from build123d import *

# Parameters (mm, degrees)
PROFILEBOSS_EXTRUDE1_DEPTH        = 16
MICROSWITCHHOLESKETCH3_W          = 12.85
MICROSWITCHHOLESKETCH3_H          = 12.05
MICROSWITCHHOLECUT_EXTRUDE1_DEPTH = 2.8
MICROSWITCHHOLESKETCH4_R          = 1.5
MICROSWITCHHOLECUT_EXTRUDE2_DEPTH = 3
CLAMPHOLECUT_EXTRUDE4_REACH       = 38.932
CLAMPHOLESSKETCH6_R               = 2
LONGWIRECHANNELCUT_EXTRUDE5_DEPTH = 37.932370625
CUT_EXTRUDE6_DEPTH                = 2.8
FILLET1_R                         = 2.2
FILLET2_R                         = 2.2


with BuildPart() as part:
    # ProfileSketch2 → ProfileBoss-Extrude1 (new body)
    with BuildSketch(Plane(origin=(0, 0, 0), x_dir=(1, 0, 0), z_dir=(0, 1, 0))):
        Polygon((0, 0), (0, -18), (28, -18), (28, 0), (24, 0), (24, -12), (8, -12), (8, 0), align=None)
    extrude(amount=PROFILEBOSS_EXTRUDE1_DEPTH)

    # MicroSwitchHoleSketch3 → MicroSwitchHoleCut-Extrude1 (cut)
    with BuildSketch(Plane.ZY):
        with Locations((9, 9.975)):
            Rectangle(MICROSWITCHHOLESKETCH3_W, MICROSWITCHHOLESKETCH3_H)
    extrude(amount=-MICROSWITCHHOLECUT_EXTRUDE1_DEPTH, mode=Mode.SUBTRACT)

    # MicroSwitchHoleSketch4 → MicroSwitchHoleCut-Extrude2 (cut)
    with BuildSketch(Plane.ZY.offset(-2.8)):
        with Locations((5.825, 10.95)):
            Circle(MICROSWITCHHOLESKETCH4_R)
        with Locations((12.175, 10.95)):
            Circle(MICROSWITCHHOLESKETCH4_R)
    extrude(amount=-MICROSWITCHHOLECUT_EXTRUDE2_DEPTH, mode=Mode.SUBTRACT)

    # ClampHolesSketch6 → ClampHoleCut-Extrude4 (cut, up to next)
    with BuildSketch(Plane(origin=(28, 0, 0), x_dir=(0, 0, -1), z_dir=(1, 0, 0)), mode=Mode.PRIVATE) as clampholecut_extrude4_sk1:
        with Locations((-9, 12)):
            Circle(CLAMPHOLESSKETCH6_R)
    clampholecut_extrude4_tool1 = extrude(clampholecut_extrude4_sk1.sketch, amount=-CLAMPHOLECUT_EXTRUDE4_REACH, mode=Mode.PRIVATE) & part.part
    # ClampHolesSketch6 → ClampHoleCut-Extrude4 (cut, up to next)
    with BuildSketch(Plane(origin=(28, 0, 0), x_dir=(0, 0, -1), z_dir=(1, 0, 0)), mode=Mode.PRIVATE) as clampholecut_extrude4_sk2:
        with Locations((-9, 4)):
            Circle(CLAMPHOLESSKETCH6_R)
    clampholecut_extrude4_tool2 = extrude(clampholecut_extrude4_sk2.sketch, amount=-CLAMPHOLECUT_EXTRUDE4_REACH, mode=Mode.PRIVATE) & part.part
    add(clampholecut_extrude4_tool1.solids().sort_by_distance((28, 12, 9))[0], mode=Mode.SUBTRACT)
    add(clampholecut_extrude4_tool2.solids().sort_by_distance((28, 4, 9))[0], mode=Mode.SUBTRACT)

    # LongWireChannelSketch7 → LongWireChannelCut-Extrude5 (cut, through all)
    with BuildSketch(Plane.ZY):
        Polygon((18, 2.525), (16.8, 2.525), (16.8, 3.075), (15.6, 3.075), (15.6, 0.875), (16.8, 0.875), (16.8, 1.425), (18, 1.425), align=None)
    extrude(amount=-LONGWIRECHANNELCUT_EXTRUDE5_DEPTH, mode=Mode.SUBTRACT)

    # ShortWireChannelSketch8 → Cut-Extrude6 (cut)
    with BuildSketch(Plane.ZY):
        Polygon((7.9, 3.95), (7.9, 0.875), (15.6, 0.875), (15.6, 3.075), (10.1, 3.075), (10.1, 3.95), align=None)
    extrude(amount=-CUT_EXTRUDE6_DEPTH, mode=Mode.SUBTRACT)

    # Fillet1
    fillet1_edges = [part.edges().sort_by_distance(p)[0] for p in [
        (2.8, 1.975, 15.6),
    ]]
    fillet(fillet1_edges, radius=FILLET1_R)

    # Fillet2
    fillet2_edges = [part.edges().sort_by_distance(p)[0] for p in [
        (28, 1.975, 15.6),
    ]]
    fillet(fillet2_edges, radius=FILLET2_R)


solid = part.part
Model file for the job. Use its own axes, mm. A direction names the side the tool comes from. Give positions to 0.01 mm unless a question says otherwise; leave off trailing zeros. Loops run counter-clockwise (first coordinate to the right, second up) from the corner with the lowest first, then second, coordinate; pieces in that order, holes last.
Item 1: Slice it at C-C (x = 20.75). Write the cut outline in (y, z) (3 decimals), plus the area to 3 significant figures.
Check values:
outline: (0, 12) - (16, 12) - (16, 18) - (2.525, 18) - (2.525, 16.8) - (3.075, 16.8) - (3.075, 15.6) - (0.875, 15.6) - (0.875, 16.8) - (1.425, 16.8) - (1.425, 18) - (0, 18) - close
area: 92.0 mm2
Item 2: Drill centre lines: line 1 along Y through (x, z) = (26.1, 9); line 2 along X through (y, z) = (6, 3.5); line 3 along X through (y, z) = (1.25, 6.75). Where is each one in solid material? Low to high.
Check values:
line 1: y = 0 to 2, 6 to 10, 14 to 16
line 2: x = 2.8 to 8, 24 to 28
line 3: x = 0 to 8, 24 to 28
Item 3: Slice it at A-A (z = 9). Write the cut outline in (x, y) (3 decimals), plus the area to 3 significant figures.
Check values:
outline: (0, 0) - (8, 0) - (8, 16) - (2.8, 16) - (2.8, 0.875) - (0, 0.875) - close; (24, 0) - (28, 0) - (28, 2) - (24, 2) - close; (24, 6) - (28, 6) - (28, 10) - (24, 10) - close; (24, 14) - (28, 14) - (28, 16) - (24, 16) - close
area: 118 mm2
Item 4: Drop flat-ended pins along their axis: P1, Ø2.5, axis at y = 12, z = 9, coming from the -X side; P2, Ø2, axis at x = 14.5, y = 12, coming from the -Z side; P3, Ø1.4, axis at x = 1, z = 5, coming from the +Y side. Give the stop position or say it passes through.
Check values:
P1: stops at x = 2.8
P2: stops at z = 12
P3: stops at y = 3.95
Item 5: Slice it at D-D (z = 5). Write the cut outline in (x, y), plus the area to 3 significant figures.
Check values:
outline: (0, 0) - (8, 0) - (8, 16) - (2.8, 16) - (2.8, 12.2) - (5.8, 12.2) - (5.8, 9.7) - (2.8, 9.7) - (2.8, 3.95) - (0, 3.95) - close; (24, 0) - (28, 0) - (28, 16) - (24, 16) - close
area: 151 mm2
Item 6: Which spindle directions (+Z, -Z, +X, -X, +Y, -Y) get a long thin tool onto all of the face, cutting with end or side? Do faces 4 (the face through (14, 2.525, 17)), 5 (the face through (4.279, 10.375, 13.561)), 6 (the face through (1, 2, 7.9)), 7 (the face through (26, 2, 9)). Say none if no direction does.
Check values:
face 4: +Z, +X, -X
face 5: -X
face 6: -X, +Y
face 7: +X
Item 7: Mould opens along X. For faces 1 (the face through (26, 14, 9)), 2 (the face through (5.8, 11, 6)), 3 (the face through (24, 8, 6)) say: +X half, -X half, draft (parallel to the pull), parting line (faces both ways), or undercut.
Check values:
face 1: draft
face 2: -X half
face 3: undercut
Item 8: Slice it at B-B (y = 10.95). Write the cut outline in (x, z) (3 decimals), plus the area to 3 significant figures.
Check values:
outline: (0, 0) - (8, 0) - (8, 12) - (24, 12) - (24, 10.702) - (28, 10.702) - (28, 18) - (0, 18) - (0, 15.425) - (2.8, 15.425) - (2.8, 13.675) - (5.8, 13.675) - (5.8, 10.675) - (2.8, 10.675) - (2.8, 7.325) - (5.8, 7.325) - (5.8, 4.325) - (2.8, 4.325) - (2.8, 2.575) - (0, 2.575) - close; (24, 0) - (28, 0) - (28, 7.298) - (24, 7.298) - close
area: 244 mm2
